Read the model definition and answer for the solid it produces. Units are mm, in the model's axes. Face numbers are marked on the shaded views. A direction names the side the tool comes from. Give positions to 0.01 mm unless a question says otherwise; leave off trailing zeros. Order: outer loops, then holes, each group sorted by start corner. A loop starts at its lowest first (then second) coordinate and runs counter-clockwise, first axis right, second up. Notation, with made-up numbers: (-12.75, 5.25) - (4.25, 5.25) arc R21 ccw to (4.25, 43.25) - close; hole circle Ø10 at (29.5, -10). An arc over 180 degrees is marked (long way). Write item = value, one per line.
```python
from build123d import *

# Parameters (mm, degrees)
CROQUIS1_W              = 46
CROQUIS1_H              = 28
SALIENTE_EXTRUIR1_DEPTH = 2
CROQUIS2_W              = 46
CROQUIS2_H              = 28
CROQUIS2_W_2            = 30
CROQUIS2_H_2            = 18
SALIENTE_EXTRUIR2_DEPTH = 16
CROQUIS3_R              = 1.75
AGUJEROS_DEPTH          = 18
CROQUIS5_W              = 6
CROQUIS5_H              = 14
CORTAR_BORDES_DEPTH     = 41.459856648
CROQUIS6_W              = 14
CROQUIS6_H              = 2
CORTAR_EXTRUIR3_DEPTH   = 47.043457733


with BuildPart() as part:
    # Croquis1 → Saliente-Extruir1 (new body)
    with BuildSketch(Plane.XY):
        Rectangle(CROQUIS1_W, CROQUIS1_H)
    extrude(amount=SALIENTE_EXTRUIR1_DEPTH)

    # Croquis2 → Saliente-Extruir2 (add)
    with BuildSketch(Plane.XY.offset(2)):
        Rectangle(CROQUIS2_W, CROQUIS2_H)
        Rectangle(CROQUIS2_W_2, CROQUIS2_H_2, mode=Mode.SUBTRACT)
    extrude(amount=SALIENTE_EXTRUIR2_DEPTH)

    # Croquis3 → Agujeros (cut)
    with BuildSketch(Plane(origin=(0, 0, 0), x_dir=(-1, 0, 0), z_dir=(0, 0, -1))):
        with Locations((-20, 0)):
            Circle(CROQUIS3_R)
        with Locations((20, 0)):
            Circle(CROQUIS3_R)
    extrude(amount=-AGUJEROS_DEPTH, mode=Mode.SUBTRACT)

    # Croquis5 → Cortar bordes (cut, through all)
    with BuildSketch(Plane.XZ.offset(14)):
        with Locations((-20, 7)):
            Rectangle(CROQUIS5_W, CROQUIS5_H)
        with Locations((20, 7)):
            Rectangle(CROQUIS5_W, CROQUIS5_H)
    extrude(amount=-CORTAR_BORDES_DEPTH, mode=Mode.SUBTRACT)

    # Croquis6 → Cortar-Extruir3 (cut, through all)
    with BuildSketch(Plane(origin=(17, 0, 0), x_dir=(0, 0, -1), z_dir=(1, 0, 0))):
        with Locations((-7, 13)):
            Rectangle(CROQUIS6_W, CROQUIS6_H)
        with Locations((-7, -13)):
            Rectangle(CROQUIS6_W, CROQUIS6_H)
    extrude(amount=-CORTAR_EXTRUIR3_DEPTH, mode=Mode.SUBTRACT)


solid = part.part
```
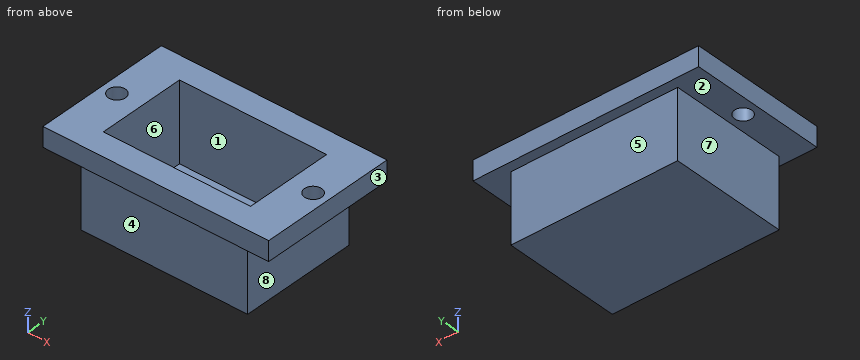
1. Section A-A (y = 0) is taken. Determine the outline of the cut face in (x, z), and give its area (3 significant figures).
Recorded:
outline = (-23, 14) - (-21.75, 14) - (-21.75, 18) - (-23, 18) - close; (-18.25, 14) - (-17, 14) - (-17, 0) - (17, 0) - (17, 14) - (18.25, 14) - (18.25, 18) - (15, 18) - (15, 2) - (-15, 2) - (-15, 18) - (-18.25, 18) - close; (21.75, 14) - (23, 14) - (23, 18) - (21.75, 18) - close
area = 152 mm^2
2. Section B-B (z = 15.5) is taken. Determine the outline of the cut face in (x, y).
Recorded:
outline = (-23, -14) - (23, -14) - (23, 14) - (-23, 14) - close; hole circle Ø3.5 at (-20, 0); hole (-15, -9) - (15, -9) - (15, 9) - (-15, 9) - close; hole circle Ø3.5 at (20, 0)
3. Section D-D (x = -5) is taken. Determine the outline of the cut face in (y, z), and give its area (3 significant figures).
Recorded:
outline = (-14, 14) - (-12, 14) - (-12, 0) - (12, 0) - (12, 14) - (14, 14) - (14, 18) - (9, 18) - (9, 2) - (-9, 2) - (-9, 18) - (-14, 18) - close
area = 160 mm^2
4. Determine the mould class of the marked faces 1, 2 and 3 for opening direction X: +X half, -X half, draft (parallel to the pull), parting line (faces both ways), or undercut.
Recorded:
face_1 = undercut
face_2 = draft
face_3 = +X half
5. Section C-C (x = 20) is taken. Determine the outline of the cut face in (y, z), and give its area (3 significant figures).
Recorded:
outline = (-14, 14) - (-1.75, 14) - (-1.75, 18) - (-14, 18) - close; (1.75, 14) - (14, 14) - (14, 18) - (1.75, 18) - close
area = 98.0 mm^2
6. For the marked faces 4, 5, 6, 7 and 8, determine the directions among +Z, -Z, +X, -X, +Y, -Y from which every point of the face is accessible in a straight line to the end or side of a thin tool.
Recorded:
face_4 = -Z, +X, -X, -Y
face_5 = -Z, +X, -X, +Y
face_6 = +Z
face_7 = -Z, -X, +Y, -Y
face_8 = -Z, +X, +Y, -Y
7. Flat-ended cylindrical pins translate along their axes: pin 1 (10 mm diameter, centred on x = -9.5, y = 3, fed in from +Z); pin 2 (2 mm diameter, centred on y = 5.5, z = 9.5, fed in from -X); pin 3 (8 mm diameter, centred on x = -2.5, z = 8, fed in from -Y); pin 4 (1 mm diameter, centred on x = -18, z = 7, fed in from +Y). Find the tip coordinate at first contact, or state that the pin passes through.
Recorded:
pin_1 = 2
pin_2 = -17
pin_3 = -12
pin_4 = through
8. Straight lines are drawn through the part: L1, parallel to X at y = -4, z = 5.5; L2, parallel to Y at x = -9, z = 3.5; L3, parallel to X at y = 1, z = 17. For each, find the intervals that lie inside material, in ascending order. Write a range as [from, to].
Recorded:
L1 = [-17, -15], [15, 17]
L2 = [-12, -9], [9, 12]
L3 = [-23, -21.44], [-18.56, -15], [15, 18.56], [21.44, 23]
